```python
from build123d import *

# Parameters (mm, degrees)
SKETCH1_W           = 370
SKETCH1_H           = 150
BOSS_EXTRUDE1_DEPTH = 15
SKETCH2_R           = 5
CUT_EXTRUDE1_DEPTH  = 30
SKETCH3_R           = 5
CUT_EXTRUDE2_DEPTH  = 30
SKETCH4_R           = 10
CUT_EXTRUDE3_DEPTH  = 16


with BuildPart() as part:
    # Sketch1 → Boss-Extrude1 (new body)
    with BuildSketch(Plane.XY):
        Rectangle(SKETCH1_W, SKETCH1_H)
    extrude(amount=BOSS_EXTRUDE1_DEPTH)

    # Sketch2 → Cut-Extrude1 (cut)
    with BuildSketch(Plane.ZY.offset(185)):
        with Locations((7.5, 61)):
            Circle(SKETCH2_R)
        with Locations((7.5, -61)):
            Circle(SKETCH2_R)
    extrude(amount=-CUT_EXTRUDE1_DEPTH, mode=Mode.SUBTRACT)

    # Sketch3 → Cut-Extrude2 (cut)
    with BuildSketch(Plane(origin=(185, 0, 0), x_dir=(0, 0, -1), z_dir=(1, 0, 0))):
        with Locations((-7.5, 61)):
            Circle(SKETCH3_R)
        with Locations((-7.5, -61)):
            Circle(SKETCH3_R)
    extrude(amount=-CUT_EXTRUDE2_DEPTH, mode=Mode.SUBTRACT)

    # Sketch4 → Cut-Extrude3 (cut, through all)
    with BuildSketch(Plane.XY.offset(15)):
        Circle(SKETCH4_R)
    extrude(amount=-CUT_EXTRUDE3_DEPTH, mode=Mode.SUBTRACT)


solid = part.part
```
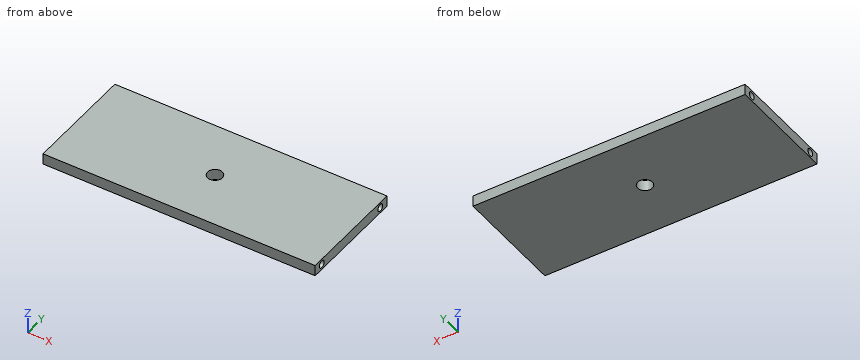
Input: part model. Units: mm. Frame: model coordinates. Give positions to 0.01 mm unless a question says otherwise; leave off trailing zeros. Order: outer loops, then holes, each group sorted by start corner. A loop starts at its lowest first (then second) coordinate and runs counter-clockwise, first axis right, second up. Notation, with made-up numbers: M -40,9.25 L -15,9.25 A6 cw -15,17.25 Z; hole C 67.5,37 d7. An arc over 180 degrees is marked long. One line per question, with ' | ' between items. Start each with the question number.
1. Material intervals for probe 1 along Y at (x, z) = (175, 7.5); probe 2 along Y at (x, z) = (0, 5.5); probe 3 along X at (y, z) = (-8, 8.75), sorted ascending. Write a range as [from, to].
2. Section query B-B (z = 7.5). Return the cut outline in (x, y).
3. First-contact query: pin 1 Ø6 at (y, z) = (-61, 7.5) entering from -X; pin 2 Ø5 at (y, z) = (-60.5, 5.5) entering from +X. Flat tips, straight axial feed; report the tip coordinate or a pass-through.
4. Section query A-A (x = 0). Return the cut outline in (y, z).
5. Section query C-C (y = 61). Return the cut outline in (x, z), and give its area (3 significant figures).
Here are the results:
1) probe 1: [-75, -66], [-56, 56], [66, 75] | probe 2: [-75, -10], [10, 75] | probe 3: [-185, -6], [6, 185]
2) outline: M -185,-75 L 185,-75 L 185,-66 L 155,-66 L 155,-56 L 185,-56 L 185,56 L 155,56 L 155,66 L 185,66 L 185,75 L -185,75 L -185,66 L -155,66 L -155,56 L -185,56 L -185,-56 L -155,-56 L -155,-66 L -185,-66 Z; hole C 0,0 d20
3) pin 1: x = -155 | pin 2: x = 155
4) outline: M -75,0 L -10,0 L -10,15 L -75,15 Z; M 10,0 L 75,0 L 75,15 L 10,15 Z
5) outline: M -185,0 L 185,0 L 185,2.5 L 155,2.5 L 155,12.5 L 185,12.5 L 185,15 L -185,15 L -185,12.5 L -155,12.5 L -155,2.5 L -185,2.5 Z | area: 4,950 mm²
